from build123d import *


with BuildPart() as f1:
    # F0 (on Front) → F1 (revolve)
    with BuildSketch(Plane.XZ):
        with BuildLine():
            Line((4.8, 22.8), (3.7, 22.8))
            ThreePointArc((3.7, 22.8), (3.558579, 22.741421), (3.5, 22.6))
            Line((3.5, 22.6), (3.5, 7.2))
            Line((3.5, 7.2), (2, 5.7))
            Line((2, 5.7), (2, 0))
            Line((2, 0), (4.3, 0))
            Line((4.3, 0), (4.3, 1))
            Line((4.3, 1), (3.8, 1))
            Line((3.8, 1), (3.8, 2))
            Line((3.8, 2), (4.3, 2))
            Line((4.3, 2), (4.3, 3))
            Line((4.3, 3), (3.8, 3))
            Line((3.8, 3), (3.8, 4))
            Line((3.8, 4), (4.3, 4))
            Line((4.3, 4), (4.3, 5))
            Line((4.3, 5), (7.8, 5))
            Line((7.8, 5), (7.8, 7.8))
            ThreePointArc((7.8, 7.8), (7.741421, 7.941421), (7.6, 8))
            Line((7.6, 8), (5.5, 8))
            ThreePointArc((5.5, 8), (5.146447, 8.146447), (5, 8.5))
            Line((5, 8.5), (5, 22.6))
            ThreePointArc((5, 22.6), (4.941421, 22.741421), (4.8, 22.8))
        make_face()
    revolve(axis=Axis((0, 0, 11.4), (0, 0, 1)))


solid = f1.part
The listing builds one solid part. Answer for the finished solid, in the listing's coordinates (mm). A direction names the side the tool comes from. Give positions to 0.01 mm unless a question says otherwise; leave off trailing zeros. Loops run counter-clockwise (first coordinate to the right, second up) from the corner with the lowest first, then second, coordinate; pieces in that order, holes last. Notation, with made-up numbers: (-26, 34.25) - (18, 34.25) arc R17 cw to (18, 66.25) - close; hole circle Ø10 at (-0.75, 44.5). An arc over 180 degrees is marked (long way). Write each question's results on one line, items separated by ' | '.
1. Consider probe 1 along Y at (x, z) = (0, 1.35); probe 2 along Y at (x, z) = (0, 11); probe 3 along Z at (x, y) = (-2.5, -5). Determine where each line is inside the solid, lowest interval first. Write a range as from..to.
Resolved:
probe 1: y = -3.8..-2, 2..3.8 | probe 2: y = -5..-3.5, 3.5..5 | probe 3: z = 5..8
2. For a pull along X with two mould halves and no side action, classify faces 5 (the face through (3.233, -1.341, 14.792)), 6 (the face through (-5.75, 5.27, 6.42)), 7 (the face through (1, -4, 22.8)), 8 (the face through (0, -2, 3)) as +X half, -X half, draft (parallel to the pull), parting line (faces both ways), or undercut.
Resolved:
face 5: undercut | face 6: parting line | face 7: draft | face 8: undercut
3. Find section A-A, the plane z = 3.5. Write down the section's boundary in (x, y), then the cut area to 3 significant figures.
Resolved:
outline: circle Ø7.6 at (0, 0); hole circle Ø4 at (0, 0) | area: 32.8 mm^2
4. Which of the six approach directions +Z, -Z, +X, -X, +Y, -Y give full straight-line access (tool end or side, diameter ignored) to faces 1 (the face through (-3.796, 0.167, 1.507)), 2 (the face through (-4.296, 0.189, 2.507)), 3 (the face through (-1.08, -4.88, 15.65)), 4 (the face through (-2, -1, 0))?
Resolved:
face 1: none | face 2: -Z | face 3: +Z | face 4: -Z, +X, -X, +Y, -Y
5. Flat-ended cylindrical pins translate along their axes: P1, Ø1.5, axis at x = -5, y = -2, coming from the -Z side; P2, Ø1.5, axis at x = 1.5, y = -0.5, coming from the +Z side; P3, Ø1.5, axis at y = 6, z = 17, coming from the +X side; P4, Ø3, axis at x = 3, z = 5, coming from the +Y side. Find the tip coordinate at first contact, or state that the pin passes through.
Resolved:
P1: stops at z = 5 | P2: stops at z = 6.03 | P3: passes through | P4: stops at y = 7.65
